Autodesk Inventor part; units mm, degrees
ref_plane "Start Plane" through (0, 0, -1.5322) normal (0, 0, 1) x (1, 0, 0)
ref_plane "End Plane" through (0, 0, 308.8193) normal (0, 0, 1) x (1, 0, 0)
ref_plane "Work Plane4" through (-9.2, -5.4006, 314.8045) normal (0.6032, 0.3541, 0.7147) x (0.7878, -0.1245, -0.6032)
ref_plane "Start Plane" through (0, 0, -1.5322) normal (0, 0, 1) x (1, 0, 0)
ref_plane "End Plane" through (0, 0, 308.8193) normal (0, 0, 1) x (1, 0, 0)
sketch "Sketch" plane through (0, 0, 0) normal (0, 0, 1) x (1, 0, 0)
  circle A0 centre (0, 0) radius 6.9342
  circle A1 centre (0, 0) radius 10.668
  dimension "d0" = 21.336
  dimension "d1" = 3.7338
extrude "Body" add sketch "Sketch" along normal up to surface (310.3515 mm away) from surface at -1.5322
sketch "Sketch3" plane through (0, 0, 0) normal (0, 0, 1) x (1, 0, 0)
  line L0 (0, 0) -> (10, 0)
ref_plane "Work Plane3" through (0, 0, 0) normal (0, -1, 0) x (1, 0, 0)
sketch "Sketch4" plane through (0, 0, 0) normal (0, -1, 0) x (1, 0, 0)
  line L0 (-2, -1.5322) -> (12, -1.5322)
  line L1 (-2, 308.8193) -> (12, 308.8193)
  dimension "d7" = 310.3515
ref_plane "Work Plane4" through (-9.2, -5.4006, 314.8045) normal (0.6032, 0.3541, 0.7147) x (0.7878, -0.1245, -0.6032)
split "Split1" plane through (-9.2, -5.4006, 314.8045) removes the side toward (0.6032, 0.3541, 0.7147)
ref_plane "Work Plane5" through (5.0201, -9.413, 309.2009) normal (-0.1943, 0.3643, 0.9108) x (0.9802, 0.037, 0.1943)
split "Split2" plane through (5.0201, -9.413, 309.2009) removes the side toward (-0.1943, 0.3643, 0.9108)
ref_plane "Work Plane6" through (9.6229, -4.605, 329.1254) normal (-0.8284, 0.3964, 0.3957) x (0.5083, 0.2353, 0.8284)
split "Split3" plane through (9.6229, -4.605, 329.1254) removes the side toward (-0.8284, 0.3964, 0.3957)
ref_plane "Work Plane7" through (-9.538, 4.7783, -16.9501) normal (0.7567, -0.3791, -0.5327) x (-0.2252, 0.6138, -0.7567)
split "Split4" plane through (-9.538, 4.7783, -16.9501) removes the side toward (0.7567, -0.3791, -0.5327)
ref_plane "Work Plane8" through (7.4352, -7.6501, -6.3246) normal (-0.3554, 0.3657, -0.8602) x (0.0964, 0.9297, 0.3554)
split "Split5" plane through (7.4352, -7.6501, -6.3246) removes the side toward (-0.3554, 0.3657, -0.8602)
equation "\"d0\" = G_H"
equation "\"d1\" = G_T"
equation "\"d2\" = G_L"
equation "\"G_H\" = 21.336"
equation "\"G_T\" = 3.7338"
equation "\"G_L\" = 310.35153"
equation "\"G_OFFSET_START\" = 1.53222"
equation "\"G_OFFSET_END\" = 4.45413"
equation "\"d4\" = -G_OFFSET_START"
equation "\"d5\" = G_OFFSET_END + B_L"
equation "\"B_L\" = 304.36517"
properties part number "ANSI - 1/2 x 0.147 - 12.219" material "Steel, Mild"
Read the model definition and answer for the solid it produces. Units are mm, in the model's axes. Round coordinates to 2 decimals unless told otherwise and drop trailing zeros. Write each loop counter-clockwise with the first axis right and the second up, starting at its lowest first coordinate (ties: lowest second). Pieces come first, ordered by that corner, then holes.
1. Determine the mould class of faces 1 (the face through (6.405, 2.656, 150.974)), 2 (the face through (7.81, -2.3, 298.91)), 3 (the face through (10.175, -3.204, 151.471)) for opening direction X: pulls with the +X half, pulls with the -X half, needs draft (parallel to the pull), parting line crosses it, or undercut.
2. Given pin 1 Ø4 at (y, z) = (-6.5, 150) entering from +X; pin 2 Ø11 at (x, y) = (0, 0) entering from +Z; pin 3 Ø3 at (x, z) = (7.5, 94) entering from +Y; pin 4 Ø8 at (x, y) = (-5, 5.5) entering from -Z, each flat-ended and moving along its own axis, determine where each tip first touches the part or whether it passes through.
3. The part is cut by section A-A, the plane y = 0. Determine the outline of the cut face in (x, z).
4. The part is cut by section B-B, the plane z = 251. Determine the outline of the cut face in (x, y).
5. Straight lines are drawn through the part: L1, parallel to Y at x = 0, z = 148; L2, parallel to X at y = 2.75, z = 17.5; L3, parallel to Y at x = 1, z = 228. For each, find the intervals that lie inside material, in ascending order.
Values:
1. face 1: undercut
1. face 2: pulls with the +X half
1. face 3: parting line crosses it
2. pin 1: stops at x = 9.67
2. pin 2: passes through
2. pin 3: stops at y = 8.82
2. pin 4: stops at z = 3.41
3. outline: (-10.67, 4.41) - (-6.93, 2.86) - (-6.93, 289.85) - (-10.67, 282.03) - close; (6.93, 9.85) - (10.67, 15.15) - (10.67, 295.36) - (6.93, 298.51) - close
4. outline: circle Ø21.34 at (0, 0); hole circle Ø13.87 at (0, 0)
5. L1: y = -10.67 to -6.93, 6.93 to 10.67
5. L2: x = -10.31 to -6.37, 6.37 to 10.31
5. L3: y = -10.62 to -6.86, 6.86 to 10.62
